The listing builds one solid part. Answer for the finished solid, in the listing's coordinates (mm). A direction names the side the tool comes from. Round coordinates to 2 decimals unless told otherwise and drop trailing zeros. Write each loop counter-clockwise with the first axis right and the second up, starting at its lowest first coordinate (ties: lowest second). Pieces come first, ordered by that corner, then holes. Notation, with made-up numbers: M 85,-16 L 106,-16 A18 ccw 106,19 Z; hole C 19,76.25 d4. An arc over 180 degrees is marked long. Put each result on its own line as item: value. Start each with the question number.
Autodesk Inventor part; units mm, degrees
ref_plane "YZ Plane" through (0, 0, 0) normal (1, 0, 0) x (0, 1, 0)
ref_plane "XZ Plane" through (0, 0, 0) normal (0, 1, 0) x (-1, 0, 0)
ref_plane "XY Plane" through (0, 0, 0) normal (0, 0, 1) x (1, 0, 0)
sketch "Sketch1" plane through (0, 0, 0) normal (0, 1, 0) x (-1, 0, 0)
  circle A0 centre (7.858, -16.0999) radius 70
  circle A1 centre (7.858, -16.0999) radius 35
  point P0 (0, 0)
  dimension "d0" = 140
  dimension "d1" = 70
extrude "Extrusion1" add sketch "Sketch1" along normal blind 10
sketch "Sketch2" plane through (-7.858, 10, -16.0999) normal (0, 1, 0) x (1, 0, 0)
  circle A0 centre (0, 0) radius 70
  circle A1 centre (0, 0) radius 62.5
  line L0 (0, 0) -> (69.5, 0)
  line L1 (69.5, 0) -> (69.5, 27.6538)
  line L2 (69.5, 27.6538) -> (69.5, -15.3132)
  line L3 (0, 0) -> (-69.5, 0)
  line L4 (-69.5, 0) -> (-69.5, 45.4592)
  point P0 (7.858, -16.0999)
  dimension "d4" = 125
  dimension "d14" = 140
  dimension "d19" = 69.5
  dimension "d20" = 69.5
extrude "Extrusion2" add sketch "Sketch2" along normal blind 40 contours A0 L2 L1 | L1 L0 A1 L3 L4 A0 | A0 L4 L3 A1 L0 L2
sketch "Sketch3" plane through (-7.858, 10, -16.0999) normal (0, 1, 0) x (1, 0, 0)
  circle A0 centre (0, 0) radius 42.5
  circle A1 centre (0, 0) radius 60.5
  point P0 (7.858, -16.0999)
  dimension "d7" = 85
extrude "Extrusion3" cut sketch "Sketch3" against normal blind 3
fillet "Fillet1" radius 3 1 edges at (-68.358, 7, -16.0999)
fillet "Fillet2" radius 3 1 edges at (-50.358, 7, -16.0999)
fillet "Fillet3" radius 1 2 edges at (-77.858, 50, -16.0999) (-70.358, 50, -16.0999)
fillet "Fillet4" radius 1 1 edges at (62.142, 0, -16.0999)
sketch "Sketch4" plane through (0, 0, 0) normal (0, 1, 0) x (-1, 0, 0)
  point P0 (0, 0)
sketch "Sketch5" plane through (0, 0, 0) normal (0, 0, 1) x (1, 0, 0)
  line L0 (-77.858, 1) -> (62.142, 1)
  line L1 (62.1388, 1) -> (-77.858, 49)
  line L2 (62.142, 49) -> (-77.858, 49)
  circle A0 centre (-7.8596, 25) radius 6
  point P0 (0, 0)
  dimension "d15" = 12
extrude "Extrusion4" cut sketch "Sketch5" along normal mid plane 300
properties part number "Rolamento_Inferior_Base"
Item 1: Determine the mould class of faces 1 (the flat face through (25, 10, 35)), 2 (the cylindrical face through (-0.271, 4.93, 18.068)), 3 (the flat face through (24, 0, 0)), 4 (the cylindrical face through (-2.137, 26.802, 50.06)) for opening direction Y: released by +Y, released by -Y, zero draft, split by the parting line, or undercut.
Item 2: Which of the six approach directions +Z, -Z, +X, -X, +Y, -Y give full straight-line access (tool end or side, diameter ignored) to faces 5 (the flat face through (-14, 10, 19)), 6 (the cylindrical face through (-3.243, 29.997, 53.748))?
Item 3: Flat-ended cylindrical pins translate along their axes: pin 1 (8 mm diameter, centred on y = 19, z = -37, fed in from +X); pin 2 (5 mm diameter, centred on x = -33, y = 11, fed in from +Z); pin 3 (2 mm diameter, centred on x = -40.5, y = 36, fed in from -Z); pin 4 (15.5 mm diameter, centred on x = -7.86, y = 25, fed in from -Z). Find the tip coordinate at first contact, or state that the pin passes through.
Item 4: Section B-B (y = 43) is taken. Give the vertices of the cut face in (x, z).
Item 5: Consider line 1 along Z through (x, y) = (31, 8); line 2 along Z through (x, y) = (-23, 9.5); line 3 along Y through (x, z) = (53, -4.5). Determine where each line is inside the solid, lowest interval first. Write a range as [from, to].
Item 6: Section A-A (y = 25) is taken. Give the vertices of the cut face in (x, z), and give its area (3 significant figures).
Output values:
1. face 1: released by +Y
1. face 2: zero draft
1. face 3: released by -Y
1. face 4: undercut
2. face 5: +Y
2. face 6: +Y, -Y
3. pin 1: stops at x = 60.07
3. pin 2: stops at z = 50.14
3. pin 3: stops at z = -78.54
3. pin 4: stops at z = -86.1
4. outline: C -7.86,-16.1 d140; hole C -7.86,-16.1 d125
5. line 1: z = [-74.32, -61.47], [-35.12, 2.92], [29.27, 42.12]
5. line 2: z = [-84.44, -74.63], [-55.86, -47.65], [15.46, 23.66], [42.43, 52.24]
5. line 3: y = [0, 10]
6. outline: M -13.86,-85.84 L -13.86,-78.31 A62.5 cw -13.86,46.11 L -13.86,53.64 A70 ccw Z; M -1.86,-85.84 A70 ccw -1.86,53.64 L -1.86,46.11 A62.5 cw -1.86,-78.31 Z
6. area: 2,940 mm^2
